Geometry: final body of the model. Coordinates: model frame, mm. Give positions to 0.01 mm unless a question says otherwise; leave off trailing zeros. Write each loop counter-clockwise with the first axis right and the second up, starting at its lowest first coordinate (ties: lowest second). Pieces come first, ordered by that corner, then holes.
from build123d import *

# Parameters (mm, degrees)
FILLET_1_R               = 4
CUT_EXTRUDE_3_DEPTH      = 6
PATTERN_CIRCULAR_1_COUNT = 6
FILLET_2_R               = 5
SKETCH_6_W               = 11.7
SKETCH_6_H               = 8
CUT_EXTRUDE_6_DEPTH      = 147.969384567
SKETCH_7_R               = 6
CUT_EXTRUDE_7_DEPTH      = 146.688022867
SKETCH_8_R               = 7.3005
CUT_EXTRUDE_8_DEPTH      = 201
FILLET_3_R               = 5


with BuildPart() as part:
    # Sketch 1 → Revolve 1 (revolve)
    with BuildSketch(Plane(origin=(0, 0, 0), x_dir=(1, 0, 0), z_dir=(0, 1, 0)), mode=Mode.PRIVATE) as revolve_1_sk:
        Polygon((15, 20), (30, 20), (30, 6), (70, 6), (70, 15), (100, 15), (100, -15), (70, -15), (70, -6), (30, -6), (30, -20), (15, -20), align=None)
    revolve(revolve_1_sk.sketch.rotate(Axis((0, 0, -20), (0, 0, 1)), 180), axis=Axis((0, 0, -20), (0, 0, 1)))

    # Fillet 1
    fillet_1_edges = [part.edges().sort_by_distance(p)[0] for p in [
        (30, 0, 6),
        (70, 0, 6),
        (70, 0, -6),
        (30, 0, -6),
    ]]
    fillet(fillet_1_edges, radius=FILLET_1_R)

    # Sketch 4 → Cut-Extrude 3 (cut, symmetric)
    with BuildSketch(Plane.XY):
        with BuildLine():
            Line((23.9577, 29.4953), (36.0505, 50.4402))
            ThreePointArc((36.0505, 50.4402), (53.693293556, 30.999302329), (61.709, 6))
            Line((61.709, 6), (37.5233, 6))
            ThreePointArc((37.5233, 6), (32.909086895, 18.999737966), (23.9577, 29.4953))
        make_face()
    cut_extrude_3 = extrude(amount=CUT_EXTRUDE_3_DEPTH, both=True, mode=Mode.SUBTRACT)

    # Pattern Circular 1: Cut-Extrude 3 ×6 about axis
    pattern_circular_1_axis = Axis((0, 0, 0), (0, 0, 1))
    for i in range(1, PATTERN_CIRCULAR_1_COUNT):
        add(cut_extrude_3.rotate(pattern_circular_1_axis, i * 360 / PATTERN_CIRCULAR_1_COUNT), mode=Mode.SUBTRACT)

    # Fillet 2
    fillet_2_edges = [part.edges().sort_by_distance(p)[0] for p in [
        (23.957802423, -29.496131034, 0),
        (61.707744572, -6.000548819, 0),
        (36.050652423, -50.441561642, 0),
        (37.5233, 6, 0),
        (36.0505, 50.4402, 0),
        (61.709, 6, 0),
        (-23.957802423, 29.496131034, 0),
        (-61.707744572, 6.000548819, 0),
        (-36.050652423, 50.441561642, 0),
        (13.565497577, 35.496131034, 0),
        (-25.657244572, 56.440748819, 0),
        (25.658347577, 56.441561642, 0),
        (-13.565497577, -35.496131034, 0),
        (25.657244572, -56.440748819, 0),
        (-25.658347577, -56.441561642, 0),
        (-37.5233, -6, 0),
        (-36.0505, -50.4402, 0),
        (-61.709, -6, 0),
    ]]
    fillet(fillet_2_edges, radius=FILLET_2_R)

    # Sketch 6 → Cut-Extrude 6 (cut, through all)
    with BuildSketch(Plane.XY.offset(20)):
        with Locations((24.15, 0)):
            Rectangle(SKETCH_6_W, SKETCH_6_H)
    extrude(amount=-CUT_EXTRUDE_6_DEPTH, mode=Mode.SUBTRACT)

    # Sketch 7 → Cut-Extrude 7 (cut, through all)
    with BuildSketch(Plane.XY.offset(15)):
        with Locations((92, 0)):
            Circle(SKETCH_7_R)
    extrude(amount=-CUT_EXTRUDE_7_DEPTH, mode=Mode.SUBTRACT)

    # Sketch 8 → Cut-Extrude 8 (cut, symmetric)
    with BuildSketch(Plane.XY):
        with Locations((-80, 0)):
            Circle(SKETCH_8_R)
    extrude(amount=CUT_EXTRUDE_8_DEPTH, both=True, mode=Mode.SUBTRACT)

    # Fillet 3
    fillet_3_edges = [part.edges().sort_by_distance(p)[0] for p in [
        (37.522529092, -6.000326816, 0),
        (23.9577, 29.4953, 0),
        (-37.522529092, 6.000326816, 0),
        (-13.564829092, 35.495626816, 0),
        (13.564829092, -35.495626816, 0),
        (-23.9577, -29.4953, 0),
    ]]
    fillet(fillet_3_edges, radius=FILLET_3_R)


solid = part.part
Q1. Pin query (flat end, axial travel): P1, Ø3, axis at y = -52.5, z = -12, coming from the -X side; P2, Ø3.5, axis at x = 25, z = 4.5, coming from the +Y side; P3, Ø11.5, axis at x = -80, y = 0, coming from the +Z side; P4, Ø6, axis at x = 50, z = 0.5, coming from the -Y side. Return the tip coordinate at first contact, or that it passes through.
Filled sheet:
P1: stops at x = -86.02
P2: stops at y = 97.26
P3: passes through
P4: stops at y = -88.27
Q2. Section A-A on x = -80. Output: boundary loops of the cut face in (y, z).
Filled sheet:
outline: (-60, -15) - (-7.3, -15) - (-7.3, 15) - (-60, 15) - close; (7.3, -15) - (60, -15) - (60, 15) - (7.3, 15) - close
Q3. Ray query, line 1 along Y through (x, z) = (0, 13.7); line 2 along Y through (x, z) = (-27.5, 10); line 3 along Z through (x, y) = (48.5, -82). Return the intervals inside material, ascending.
Filled sheet:
line 1: y = -100 to -70, -30 to -15, 15 to 30, 70 to 100
line 2: y = -96.14 to -64.37, -11.99 to 11.99, 64.37 to 96.14
line 3: z = -15 to 15
Q4. Section D-D on y = -77. Output: boundary loops of the cut face in (x, z), plus the area to 3 significant figures.
Filled sheet:
outline: (-63.8, -15) - (63.8, -15) - (63.8, 15) - (-63.8, 15) - close
area: 3,830 mm2
Q5. Section B-B on x = 0. Count the separate pieces of the cut face and the enclosed holes in it, plus the area to 3 significant figures.
Filled sheet:
separate pieces: 4
enclosed holes: 0
area: 3,410 mm2
